from build123d import *

# Parameters (mm, degrees)
SKETCH1_W           = 25
SKETCH1_H           = 24
BOSS_EXTRUDE1_DEPTH = 1
SKETCH2_R           = 0.5
CUT_EXTRUDE1_DEPTH  = 18.356554958
SKETCH3_W           = 8.5
SKETCH3_H           = 8.5
BOSS_EXTRUDE2_DEPTH = 3.21
SKETCH4_R           = 3.876557288
BOSS_EXTRUDE3_DEPTH = 1.88


with BuildPart() as part:
    # Sketch1 → Boss-Extrude1 (new body)
    with BuildSketch(Plane(origin=(0, 0, 0), x_dir=(1, 0, 0), z_dir=(0, 1, 0))):
        Rectangle(SKETCH1_W, SKETCH1_H)
    extrude(amount=BOSS_EXTRUDE1_DEPTH)

    # Sketch2 → Cut-Extrude1 (cut, through all)
    with BuildSketch(Plane(origin=(0, 1, 0), x_dir=(1, 0, 0), z_dir=(0, 1, 0))):
        with Locations(Location((-10.5, -10, 0), (0, 0, 270))):
            Circle(SKETCH2_R)
        with Locations(Location((10.5, -10, 0), (0, 0, 90))):
            Circle(SKETCH2_R)
        with Locations(Location((-10.5, 2.5, 0), (0, 0, 270))):
            Circle(SKETCH2_R)
        with Locations(Location((10.5, 2.5, 0), (0, 0, 90))):
            Circle(SKETCH2_R)
    extrude(amount=-CUT_EXTRUDE1_DEPTH, mode=Mode.SUBTRACT)

    # Sketch3 → Boss-Extrude2 (add)
    with BuildSketch(Plane(origin=(0, 1, 0), x_dir=(1, 0, 0), z_dir=(0, 1, 0))):
        with Locations((0, 2.5)):
            Rectangle(SKETCH3_W, SKETCH3_H)
    extrude(amount=BOSS_EXTRUDE2_DEPTH)

    # Sketch4 → Boss-Extrude3 (add)
    with BuildSketch(Plane(origin=(0, 4.21, 0), x_dir=(1, 0, 0), z_dir=(0, 1, 0))):
        with Locations(Location((0, 2.5, 0), (0, 0, 270))):
            Circle(SKETCH4_R)
    extrude(amount=BOSS_EXTRUDE3_DEPTH)


solid = part.part
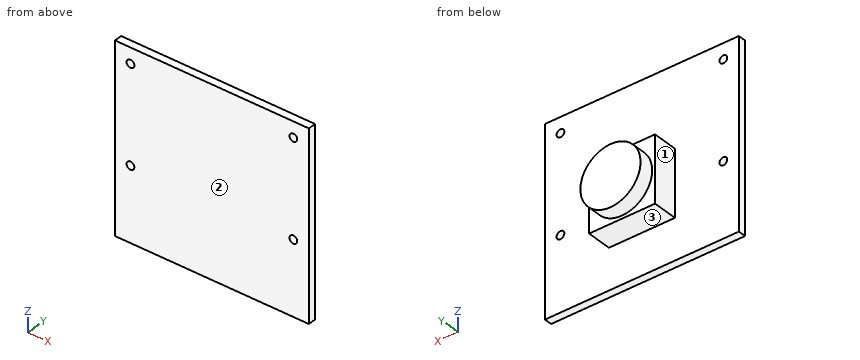
Input: part model. Units: mm. Frame: model coordinates. Face numbers are marked on the shaded views. A direction names the side the tool comes from. Give positions to 0.01 mm unless a question says otherwise; leave off trailing zeros. Write each loop counter-clockwise with the first axis right and the second up, starting at its lowest first coordinate (ties: lowest second). Pieces come first, ordered by that corner, then holes.
Q1. Material intervals for probe 1 along Z at (x, y) = (10.5, 0.75); probe 2 along X at (y, z) = (0.35, 10); probe 3 along Y at (x, z) = (-6.25, -1.5), sorted ascending.
Q2. Section C-C, the plane z = -2.5. Output: boundary loops of the cut face in (x, y), plus the area to 3 significant figures.
Q3. Set-up query: the marked faces 1, 2 and 3. Return all of +Z, -Z, +X, -X, +Y, -Y with unobstructed straight access to the full face (end or side cutting, diameter ignored); none if empty.
Q4. Section D-D, the plane y = 3.25. Output: boundary loops of the cut face in (x, z).
Q5. Section A-A, the plane z = 10. Output: boundary loops of the cut face in (x, y).
Q6. First-contact query: P1, Ø2.5, axis at x = -1.5, y = 3, coming from the +Z side; P2, Ø2, axis at y = 3.5, z = -3, coming from the -X side; P3, Ø3.5, axis at y = 3.5, z = -3, coming from the +X side; P4, Ø4, axis at x = 6.5, z = 6, coming from the -Y side. Flat tips, straight axial feed; report the tip coordinate or a pass-through.
Q7. Section B-B, the plane x = 0. Output: boundary loops of the cut face in (y, z).
Filled in:
1. probe 1: z = -12 to -3, -2 to 9.5, 10.5 to 12
1. probe 2: x = -12.5 to -11, -10 to 10, 11 to 12.5
1. probe 3: y = 0 to 1
2. outline: (-12.5, 0) - (-11, 0) - (-11, 1) - (-12.5, 1) - close; (-10, 0) - (10, 0) - (10, 1) - (4.25, 1) - (4.25, 4.21) - (3.88, 4.21) - (3.88, 6.09) - (-3.88, 6.09) - (-3.88, 4.21) - (-4.25, 4.21) - (-4.25, 1) - (-10, 1) - close; (11, 0) - (12.5, 0) - (12.5, 1) - (11, 1) - close
2. area: 64.9 mm2
3. face 1: +Z, -Z, -X, +Y
3. face 2: +Z, -Z, +X, -X, -Y
3. face 3: -Z, +X, -X, +Y
4. outline: (-4.25, -6.75) - (4.25, -6.75) - (4.25, 1.75) - (-4.25, 1.75) - close
5. outline: (-12.5, 0) - (-11, 0) - (-11, 1) - (-12.5, 1) - close; (-10, 0) - (10, 0) - (10, 1) - (-10, 1) - close; (11, 0) - (12.5, 0) - (12.5, 1) - (11, 1) - close
6. P1: stops at z = 1.75
6. P2: stops at x = -4.25
6. P3: stops at x = 4.25
6. P4: stops at y = 0
7. outline: (0, -12) - (1, -12) - (1, -6.75) - (4.21, -6.75) - (4.21, -6.38) - (6.09, -6.38) - (6.09, 1.38) - (4.21, 1.38) - (4.21, 1.75) - (1, 1.75) - (1, 12) - (0, 12) - close
